The drawing under review shows one solid part. Ordinate dimensions are in mm from its lowest x, y, z. Round coordinates to 2 decimals unless told otherwise and drop trailing zeros. Write each loop counter-clockwise with the first axis right and the second up, starting at its lowest first coordinate (ties: lowest second). Pieces come first, ordered by that corner, then holes. Notation, with made-up numbers: (49.5, -31.5) - (80.5, -31.5) arc R30 ccw to (80.5, 1.5) - close; hole circle Ø4 at (-11.5, -29). An arc over 180 degrees is marked (long way). Answer in a Markdown table with one row per item. Add a question column.
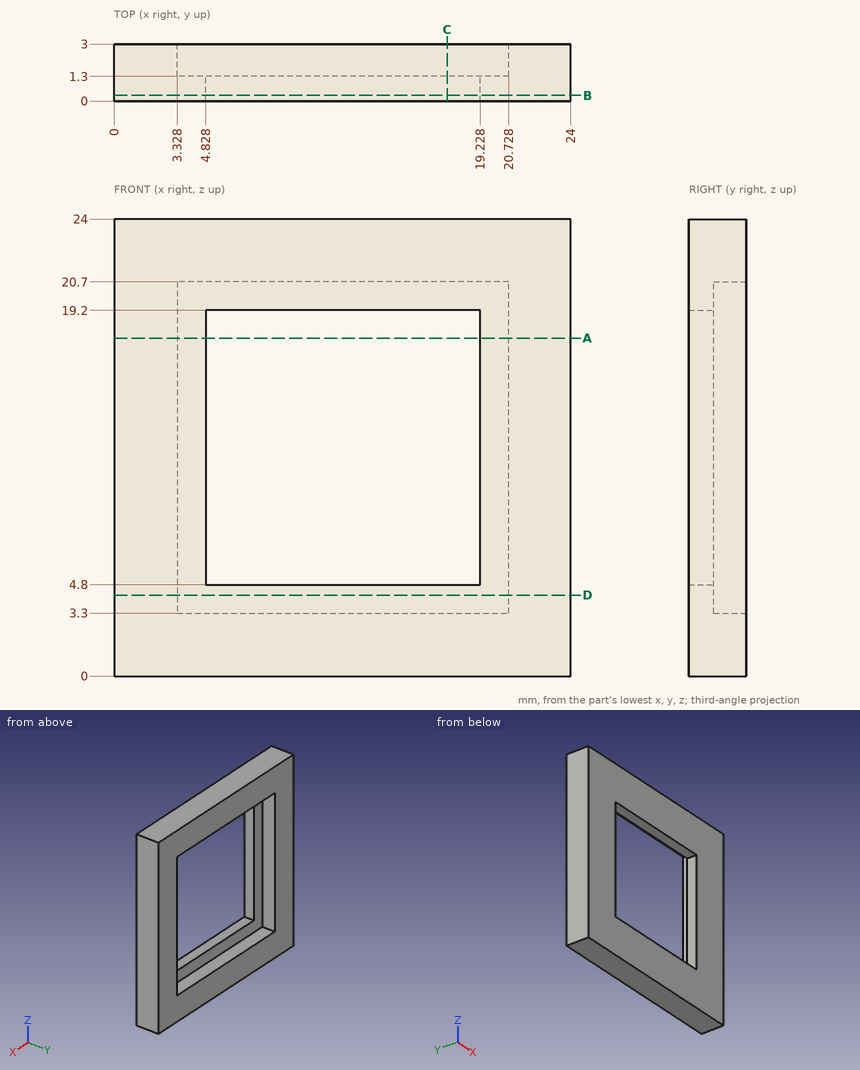
Q1. Add section C-C on x = 17.5. State the section outline as (y, z) points.
Q2. Add section A-A on z = 17.75. State the section outline as (x, y) points, then the cut area to 3 significant figures.
Q3. Insertion check: pin 1 Ø8 at (x, z) = (11, 13) entering from -Y. The pin has a flat end and moves straight along its axis. Give the tip position at first contact, or say it passes through.
Q4. To check wall thickness, follow probe 1 along Z at (x, y) = (8.75, 2.65); probe 2 along X at (y, z) = (0.55, 6); probe 3 along X at (y, z) = (1.95, 7). State the ranges of each line that lie inside material, in increasing order.
Q5. Add section D-D on z = 4.25. State the section outline as (x, y) points.
Q6. Add section B-B on y = 0.3. State the section outline as (x, z) points, then the cut area to 3 significant figures.
Answer sheet:
| question | item | result |
|---|---|---|
| 1 | outline | (0, 0) - (3, 0) - (3, 3.3) - (1.3, 3.3) - (1.3, 4.8) - (0, 4.8) - close; (0, 19.2) - (1.3, 19.2) - (1.3, 20.7) - (3, 20.7) - (3, 24) - (0, 24) - close |
| 2 | outline | (0, 0) - (4.83, 0) - (4.83, 1.3) - (3.33, 1.3) - (3.33, 3) - (0, 3) - close; (19.23, 0) - (24, 0) - (24, 3) - (20.73, 3) - (20.73, 1.3) - (19.23, 1.3) - close |
| 2 | area | 23.7 mm² |
| 3 | pin 1 | passes through |
| 4 | probe 1 | z = 0 to 3.3, 20.7 to 24 |
| 4 | probe 2 | x = 0 to 4.83, 19.23 to 24 |
| 4 | probe 3 | x = 0 to 3.33, 20.73 to 24 |
| 5 | outline | (0, 0) - (24, 0) - (24, 3) - (20.73, 3) - (20.73, 1.3) - (3.33, 1.3) - (3.33, 3) - (0, 3) - close |
| 6 | outline | (0, 0) - (24, 0) - (24, 24) - (0, 24) - close; hole (4.83, 4.8) - (19.23, 4.8) - (19.23, 19.2) - (4.83, 19.2) - close |
| 6 | area | 369 mm² |
